from build123d import *

# Parameters (mm, degrees)
SKETCH1_W                = 10
SKETCH1_H                = 12.5
BOSS_EXTRUDE1_DEPTH      = 22.5
BOSS_EXTRUDE1_DEPTH_BACK = 22.5
SKETCH2_W                = 10
SKETCH2_H                = 38.75
BOSS_EXTRUDE2_DEPTH      = 5
BOSS_EXTRUDE2_DEPTH_BACK = 5
F_6_CLEARANCE_HOLE1_D    = 3.7973
BOSS_EXTRUDE5_DEPTH      = 8
FILLET2_R                = 5


with BuildPart() as part:
    # Sketch1 → Boss-Extrude1 (new body, two sides)
    with BuildSketch(Plane(origin=(0, 0, 0), x_dir=(0, 0, -1), z_dir=(1, 0, 0))) as boss_extrude1_sk:
        with Locations((12.5, 0)):
            Rectangle(SKETCH1_W, SKETCH1_H)
    extrude(amount=BOSS_EXTRUDE1_DEPTH)
    extrude(boss_extrude1_sk.sketch, amount=-BOSS_EXTRUDE1_DEPTH_BACK)

    # Sketch2 → Boss-Extrude2 (add, two sides)
    with BuildSketch(Plane(origin=(0, 0, 0), x_dir=(0, 0, -1), z_dir=(1, 0, 0))) as boss_extrude2_sk:
        with Locations((12.5, -25.625)):
            Rectangle(SKETCH2_W, SKETCH2_H)
    extrude(amount=BOSS_EXTRUDE2_DEPTH)
    extrude(boss_extrude2_sk.sketch, amount=-BOSS_EXTRUDE2_DEPTH_BACK)

    # 6 Clearance Hole1 (through all)
    with Locations(Plane(origin=(0, 0, -17.5), x_dir=(-1, 0, 0), z_dir=(0, 0, -1))):
        with Locations((16.5, 0), (-16.5, 0)):
            Hole(F_6_CLEARANCE_HOLE1_D / 2)

    # Sketch3 → Boss-Extrude5 (add)
    with BuildSketch(Plane(origin=(0, 4.290110382, -45.957658497), x_dir=(-1, 0, 0), z_dir=(0, 0.5, 0.866025404))):
        Polygon((50, 53.165316994), (50, 65.665316994), (6.25, 65.665316994), (6.25, 116.915316994), (-6.25, 116.915316994), (-6.25, 65.665316994), (-50, 65.665316994), (-50, 53.165316994), (-6.25, 53.165316994), (-6.25, 1.915316994), (6.25, 1.915316994), (6.25, 53.165316994), align=None)
    extrude(amount=BOSS_EXTRUDE5_DEPTH)

    # Fillet2
    fillet2_edges = [part.edges().sort_by_distance(p)[0] for p in [
        (0, -29, -17.5),
    ]]
    fillet(fillet2_edges, radius=FILLET2_R)


solid = part.part
Build history of the part. All positions in model axes, mm. A direction names the side the tool comes from. Coordinates: 2 decimals unless noted, no trailing zeros. Order: outer loops, then holes, each group sorted by start corner. A loop starts at its lowest first (then second) coordinate and runs counter-clockwise, first axis right, second up. Notation, with made-up numbers: (-6.75, -39) -> (15.25, -39) arc R17 ccw to (15.25, -29) -> close; hole circle Ø4 at (63.25, 47.25). An arc over 180 degrees is marked (long way). One line per item, written item: value.
(1) Slice it at D-D, the plane z = -11. List the corners of the cut face in (x, y), plus the area to 3 significant figures.
Checked values:
outline: (-50, -51.35) -> (-6.25, -51.35) -> (-6.25, -56.26) -> (6.25, -56.26) -> (6.25, -51.35) -> (50, -51.35) -> (50, -40.26) -> (5, -40.26) -> (5, -6.25) -> (22.5, -6.25) -> (22.5, 6.25) -> (-22.5, 6.25) -> (-22.5, -6.25) -> (-5, -6.25) -> (-5, -40.26) -> (-50, -40.26) -> close; hole circle Ø3.8 at (-16.5, 0); hole circle Ø3.8 at (16.5, 0)
area: 2,050 mm2
(2) Slice it at B-B, the plane y = -8.5. List the corners of the cut face in (x, z).
Checked values:
outline: (-6.25, -38.57) -> (6.25, -38.57) -> (6.25, -29.34) -> (-6.25, -29.34) -> close; (-5, -17.5) -> (5, -17.5) -> (5, -7.5) -> (-5, -7.5) -> close
(3) Tool access for faces 4 (the flat face through (27.8, -50.6, -9.7)), 5 (the flat face through (22.5, 0, -12)), 6 (the flat face through (-28.4, -50.6, -9.7)), 7 (the flat face through (-22.5, 0, -12)), 8 (the flat face through (-5, -21, -13)): list every direction of +Z, -Z, +X, -X, +Y, -Y with a clear straight run to the whole face (end or side of a thin tool).
Checked values:
face 4: +Z, +X, -Y
face 5: +Z, -Z, +X, +Y
face 6: +Z, -X, -Y
face 7: +Z, -Z, -X, +Y
face 8: +Z, -X
(4) Drop flat-ended pins along their axis: pin 1 Ø3 at (x, z) = (-2, -10) entering from +Y; pin 2 Ø12 at (x, y) = (4.5, -42.5) entering from +Z; pin 3 Ø6 at (y, z) = (-27.5, -16) entering from +X. Give the stop position or say it passes through.
Checked values:
pin 1: y = 6.25
pin 2: z = -6.24
pin 3: x = 6.25
(5) Mould opens along Y. For faces 1 (the flat face through (-3.47, -47.086, -7.058)), 2 (the flat face through (50, -45, -13)), 3 (the flat face through (0.087, 4.603, -41.584)) say: pulls with the +Y half, pulls with the -Y half, needs draft (parallel to the pull), parting line crosses it, or undercut.
Checked values:
face 1: undercut
face 2: needs draft
face 3: pulls with the +Y half
(6) Slice it at C-C, the plane x = 1. List the corners of the cut face in (y, z).
Checked values:
outline: (-96.96, 12.5) -> (2.63, -45) -> (6.63, -38.07) -> (-12.84, -26.83) arc R5 cw to (-10.34, -17.5) -> (6.25, -17.5) -> (6.25, -7.5) -> (-45, -7.5) -> (-45, -8.26) -> (-92.96, 19.43) -> close
(7) Probe line 1 (Y direction, x = 16.5, z = -12.5); line 2 (Y direction, x = 16.5, z = -13.5); line 3 (X direction, y = -11.5, z = -14.5). List the from-to ranges inside material, lowest first. Write a range as [from, to].
Checked values:
line 1: [-52.22, -37.78], [-6.25, -1.9], [1.9, 6.25]
line 2: [-51.93, -38.36], [-6.25, -1.9], [1.9, 6.25]
line 3: [-5, 5]
(8) Slice it at A-A, the plane x = -16.5. List the corners of the cut face in (y, z) (3 decimals).
Checked values:
outline: (-52.578, -13.125) -> (-41.752, -19.375) -> (-37.752, -12.447) -> (-48.578, -6.197) -> close; (-6.25, -17.5) -> (-1.899, -17.5) -> (-1.899, -7.5) -> (-6.25, -7.5) -> close; (1.899, -17.5) -> (6.25, -17.5) -> (6.25, -7.5) -> (1.899, -7.5) -> close
